Check sheet for the modelled part. Datum: model origin and axes. Units: mm. Face numbers are marked on the shaded views. Round coordinates to 2 decimals unless told otherwise and drop trailing zeros. Write each loop counter-clockwise with the first axis right and the second up, starting at its lowest first coordinate (ties: lowest second). Pieces come first, ordered by that corner, then holes. Notation, with made-up numbers: (-38.5, 23) -> (-24.5, 23) arc R14 ccw to (-24.5, 39) -> close; hole circle Ø1 at (85.25, 37.5). An arc over 180 degrees is marked (long way). One line per item, written item: value. Start each with the question number.
```python
from build123d import *

# Parameters (mm, degrees)
F0_R      = 11
F1_DEPTH  = 40
F3_DEPTH  = 35
F6_DEPTH  = 7.501
F8_DEPTH  = 7.501
F5_R      = 8
F9_DEPTH  = 25
F10_R     = 2.5
F11_DEPTH = 7.501
F12_R     = 2.5
F13_DEPTH = 7.5010001
F14_SIZE  = 2
F17_DEPTH = 4.5010001
F19_R     = 4
F20_DEPTH = 4.5010001


with BuildPart() as f1:
    # F0 (on Top) → F1 (new body)
    with BuildSketch(Plane.XY):
        Circle(F0_R)
    extrude(amount=F1_DEPTH)

    # F2 (on face) → F3 (cut)
    with BuildSketch(Plane.XY.offset(40)):
        with BuildLine():
            ThreePointArc((-3.5, -10.4283268073), (0, -11), (3.5, -10.4283268073))
            Line((3.5, -10.4283268073), (3.5, 10.4283268073))
            ThreePointArc((3.5, 10.4283268073), (0, 11), (-3.5, 10.4283268073))
            Line((-3.5, 10.4283268073), (-3.5, -10.4283268073))
        make_face()
    extrude(amount=-F3_DEPTH, mode=Mode.SUBTRACT)

    # F4 (on face) → F6 (cut, through all)
    with BuildSketch(Plane.YZ.offset(-3.5)):
        Polygon((-10.4283268073, 35), (0, 40), (-10.4283268073, 40), align=None)
    extrude(amount=-F6_DEPTH, mode=Mode.SUBTRACT)

    # F7 (on face) → F8 (cut, through all)
    with BuildSketch(Plane(origin=(3.5, 0, 0), x_dir=(0, -1, 0), z_dir=(-1, 0, 0))):
        Polygon((10.4283268073, 40), (0, 40), (10.4283268073, 35), align=None)
    extrude(amount=-F8_DEPTH, mode=Mode.SUBTRACT)

    # F5 (on face) → F9 (join)
    with BuildSketch(Plane(origin=(0, 0, 0), x_dir=(1, 0, 0), z_dir=(0, 0, -1))):
        Circle(F5_R)
    extrude(amount=F9_DEPTH)

    # F10 (on face) → F11 (cut, through all)
    with BuildSketch(Plane(origin=(3.5, 0, 0), x_dir=(0, -1, 0), z_dir=(-1, 0, 0))):
        with Locations((0, 25)):
            Circle(F10_R)
    extrude(amount=-F11_DEPTH, mode=Mode.SUBTRACT)

    # F12 (on face) → F13 (cut, through all)
    with BuildSketch(Plane.YZ.offset(-3.5)):
        with Locations((0, 25)):
            Circle(F12_R)
    extrude(amount=-F13_DEPTH, mode=Mode.SUBTRACT)

    # F14
    f14_edges = [f1.edges().sort_by_distance(p)[0] for p in [
        (-8, 0, -25),
    ]]
    chamfer(f14_edges, length=F14_SIZE)

    # F16 (on offset) → F17 (cut, through all)
    with BuildSketch(Plane.YZ.offset(-6.5)):
        with BuildLine():
            ThreePointArc((1.9999999297, 21.7011209295), (3.4641015949, 23.1652225501), (4, 25.1652225852))
            ThreePointArc((4, 25.1652225852), (3.4641016169, 27.1652225821), (2.0000000062, 28.6293241968))
            ThreePointArc((2.0000000062, 28.6293241968), (7.14e-08, 29.1652225852), (-1.9999998825, 28.6293242682))
            ThreePointArc((-1.9999998825, 28.6293242682), (-3.4641015812, 27.165222644), (-4, 25.1652225852))
            ThreePointArc((-4, 25.1652225852), (-3.4641016169, 23.1652225883), (-2.0000000062, 21.7011209736))
            ThreePointArc((-2.0000000062, 21.7011209736), (-4.42e-08, 21.1652225852), (1.9999999297, 21.7011209295))
        make_face()
        with BuildLine():
            Line((4, 22.8558215084), (4, 25.1652225852))
            ThreePointArc((4, 25.1652225852), (3.4641015949, 23.1652225501), (1.9999999297, 21.7011209295))
            Line((1.9999999297, 21.7011209295), (4, 22.8558215084))
        make_face()
        with BuildLine():
            ThreePointArc((2.0000000062, 28.6293241968), (3.4641016169, 27.1652225821), (4, 25.1652225852))
            Line((4, 25.1652225852), (4, 27.474623662))
            Line((4, 27.474623662), (2.0000000062, 28.6293241968))
        make_face()
        with BuildLine():
            ThreePointArc((-1.9999998825, 28.6293242682), (7.14e-08, 29.1652225852), (2.0000000062, 28.6293241968))
            Line((2.0000000062, 28.6293241968), (0, 29.7840247387))
            Line((0, 29.7840247387), (-1.9999998825, 28.6293242682))
        make_face()
        with BuildLine():
            Line((0, 20.5464204317), (1.9999999297, 21.7011209295))
            ThreePointArc((1.9999999297, 21.7011209295), (-4.42e-08, 21.1652225852), (-2.0000000062, 21.7011209736))
            Line((-2.0000000062, 21.7011209736), (0, 20.5464204317))
        make_face()
        with BuildLine():
            ThreePointArc((-4, 25.1652225852), (-3.4641015812, 27.165222644), (-1.9999998825, 28.6293242682))
            Line((-1.9999998825, 28.6293242682), (-4, 27.474623662))
            Line((-4, 27.474623662), (-4, 25.1652225852))
        make_face()
        with BuildLine():
            Line((-4, 22.8558215084), (-2.0000000062, 21.7011209736))
            ThreePointArc((-2.0000000062, 21.7011209736), (-3.4641016169, 23.1652225883), (-4, 25.1652225852))
            Line((-4, 25.1652225852), (-4, 22.8558215084))
        make_face()
    extrude(amount=-F17_DEPTH, mode=Mode.SUBTRACT)

    # F19 (on offset) → F20 (cut, through all)
    with BuildSketch(Plane(origin=(6.5, 0, 0), x_dir=(0, -1, 0), z_dir=(-1, 0, 0))):
        with Locations((0, 25)):
            Circle(F19_R)
    extrude(amount=-F20_DEPTH, mode=Mode.SUBTRACT)


solid = f1.part
```
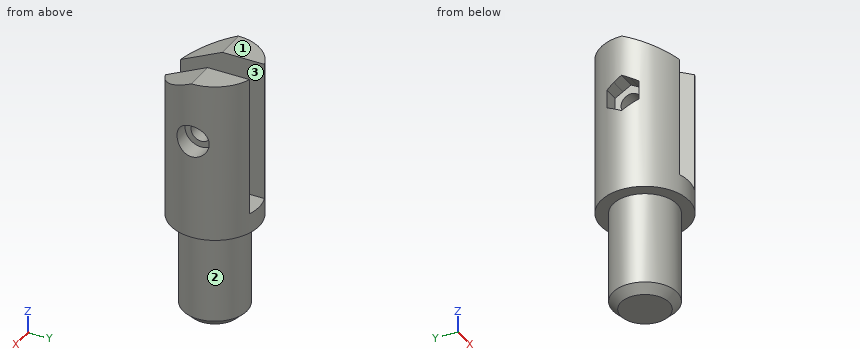
1. Material ranges on probe 1 along Z at (x, y) = (-4.2, 0); probe 2 along Z at (x, y) = (9.9, 0); probe 3 along Z at (x, y) = (8.75, 5.75), recorded low to high.
2. Release check for a two-part mould opening along X. For the marked faces 1, 2 and 3 record: +X half, -X half, draft (parallel to the pull), parting line (faces both ways), or undercut.
3. Cross-section at D-D (y = 1.25). Give the number of separate pieces and of enclosed holes in the cut face, plus the area to 3 significant figures.
4. Cross-section at C-C (x = -9.5). Record the cut outline in (y, z), plus the area to 3 significant figures.
5. Cross-section at A-A (x = 0). Record the cut outline in (y, z), plus the area to 3 significant figures.
6. Cross-section at B-B (z = 25). Record the cut outline in (x, y), plus the area to 3 significant figures.
7. Depth check by flat-ended pin: pin 1 Ø10.5 at (y, z) = (0, 25) entering from -X; pin 2 Ø4 at (y, z) = (1.5, 24.5) entering from -X; pin 3 Ø4 at (x, z) = (-9, 25) entering from +Y; pin 4 Ø6 at (x, y) = (-4.5, -4.5) entering from +Z. Enter the tip coordinate at first touch or a pass-through.
Working result:
1. probe 1: z = -25 to 22.5, 27.5 to 40
1. probe 2: z = 0 to 21, 29 to 40
1. probe 3: z = 0 to 40
2. face 1: draft
2. face 2: parting line
2. face 3: undercut
3. separate pieces: 3
3. enclosed holes: 0
3. area: 926 mm^2
4. outline: (-5.55, 0) -> (5.55, 0) -> (5.55, 40) -> (0, 40) -> (-5.55, 37.34) -> close; hole (-4, 22.86) -> (0, 20.55) -> (4, 22.86) -> (4, 27.47) -> (0, 29.78) -> (-4, 27.47) -> close
4. area: 381 mm^2
5. outline: (-11, 0) -> (-8, 0) -> (-8, -23) -> (-6, -25) -> (6, -25) -> (8, -23) -> (8, 0) -> (11, 0) -> (11, 5) -> (-11, 5) -> close
5. area: 506 mm^2
6. outline: (-10.25, -4) arc R11 ccw to (-3.5, -10.43) -> (-3.5, -2.5) -> (-6.5, -2.5) -> (-6.5, -4) -> close; (-10.25, 4) -> (-6.5, 4) -> (-6.5, 2.5) -> (-3.5, 2.5) -> (-3.5, 10.43) arc R11 ccw to start; (3.5, -10.43) arc R11 ccw to (10.25, -4) -> (6.5, -4) -> (6.5, -2.5) -> (3.5, -2.5) -> close; (3.5, 2.5) -> (6.5, 2.5) -> (6.5, 4) -> (10.25, 4) arc R11 ccw to (3.5, 10.43) -> close
6. area: 131 mm^2
7. pin 1: stops at x = -11
7. pin 2: stops at x = -6.5
7. pin 3: stops at y = 8.49
7. pin 4: stops at z = 39.28
